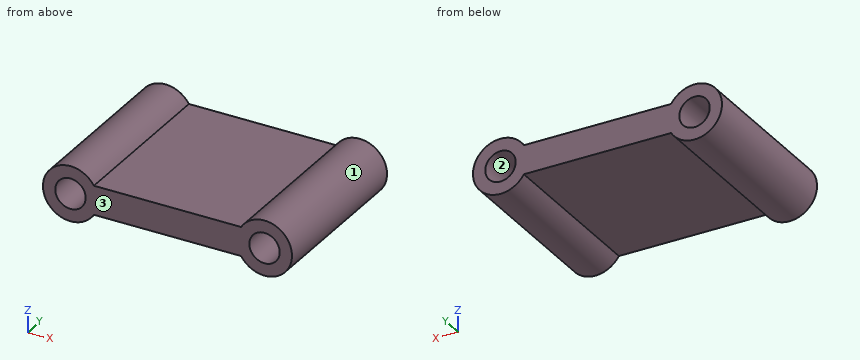
Solid Edge part; units mm, degrees
sketch "Sketch1" plane through (0, 0, 0) normal (0, -1, 0) x (1, 0, 0)
  circle A0 centre (-1.3109, 12.3912) radius 1.05
  circle A1 centre (12.0891, 12.3912) radius 1.05
  line L0 (0.3046, 13.3912) -> (10.4735, 13.3912)
  line L1 (10.4735, 11.3912) -> (0.3046, 11.3912)
  arc A2 (0.3046, 11.3912) -> (0.3046, 13.3912) centre (-1.3109, 12.3912) cw
  arc A3 (10.4735, 13.3912) -> (10.4735, 11.3912) centre (12.0891, 12.3912) cw
extrude "Protrusion1" add sketch "Sketch1" against normal blind 11.5
For this review, take the finished solid that the model builds, in its own axes (mm). Face numbers are marked on the shaded views. Coordinates: 2 decimals unless noted, no trailing zeros. Write each loop counter-clockwise with the first axis right and the second up, starting at its lowest first coordinate (ties: lowest second). Pieces come first, ordered by that corner, then holes. Notation, with made-up numbers: (78, -22) -> (104, -22) arc R16 ccw to (104, 9) -> close; hole circle Ø5 at (-39, 84). An arc over 180 degrees is marked (long way). Put each result on its own line as item: value.
Q1. Take a section at D-D, the plane y = 7.75. State the section outline as (x, z) points.
From the geometry:
outline: (0.3, 11.39) -> (10.47, 11.39) arc R1.9 ccw (long way) to (10.47, 13.39) -> (0.3, 13.39) arc R1.9 ccw (long way) to start; hole circle Ø2.1 at (-1.31, 12.39); hole circle Ø2.1 at (12.09, 12.39)
Q2. Take a section at C-C, the plane x = 11.5. State the section outline as (y, z) points, then the cut area to 3 significant figures.
From the geometry:
outline: (0, 10.58) -> (11.5, 10.58) -> (11.5, 11.52) -> (0, 11.52) -> close; (0, 13.26) -> (11.5, 13.26) -> (11.5, 14.2) -> (0, 14.2) -> close
area: 21.6 mm2
Q3. Take a section at B-B, the plane z = 13.65. State the section outline as (x, y) points, then the cut area to 3 significant figures.
From the geometry:
outline: (-2.73, 0) -> (0.11, 0) -> (0.11, 11.5) -> (-2.73, 11.5) -> close; (10.67, 0) -> (13.51, 0) -> (13.51, 11.5) -> (10.67, 11.5) -> close
area: 65.5 mm2
Q4. Clearance check with flat-ended pins moving along their axes: pin 1 Ø5 at (x, y) = (8.5, 4.5) entering from -Z; pin 2 Ø6 at (x, y) = (5, 7) entering from -Z; pin 3 Ø3 at (x, y) = (10.5, 2.5) entering from +Z. State where each tip first meets the part, or that it passes through.
From the geometry:
pin 1: stops at z = 10.83
pin 2: stops at z = 11.39
pin 3: stops at z = 14.29
Q5. The part is to be moulded in two halves that separate along Z. For the marked faces 1, 2 and 3, say which applies: +Z half, -Z half, draft (parallel to the pull), parting line (faces both ways), or undercut.
From the geometry:
face 1: parting line
face 2: undercut
face 3: draft
Q6. Take a section at A-A, the plane z = 11.95. State the section outline as (x, y) points.
From the geometry:
outline: (-3.16, 0) -> (-2.26, 0) -> (-2.26, 11.5) -> (-3.16, 11.5) -> close; (-0.36, 0) -> (11.14, 0) -> (11.14, 11.5) -> (-0.36, 11.5) -> close; (13.04, 0) -> (13.94, 0) -> (13.94, 11.5) -> (13.04, 11.5) -> close
Q7. Wall thickness on L1, parallel to X at y = 5.5, z = 12.35; L2, parallel to X at y = 4.5, z = 13.15; L3, parallel to Z at x = 7, y = 3: over which ranges is each line inside the solid? List them lowest first.
From the geometry:
L1: x = -3.21 to -2.36, -0.26 to 11.04, 13.14 to 13.99
L2: x = -3.05 to -2.04, -0.59 to 11.36, 12.81 to 13.83
L3: z = 11.39 to 13.39
